CAD build for the part. Positions are in the model's coordinates, mm. Face numbers are marked on the shaded views. A direction names the side the tool comes from. Round coordinates to 2 decimals unless told otherwise and drop trailing zeros. Order: outer loops, then holes, each group sorted by start corner. A loop starts at its lowest first (then second) coordinate and runs counter-clockwise, first axis right, second up. Notation, with made-up numbers: (74.5, 4) - (86.5, 4) arc R12 cw to (86.5, 15) - close; hole circle Ø4 at (13.5, 20). An arc over 180 degrees is marked (long way). Use one line per item in the form item = value. Start each with the question number.
Autodesk Inventor part; units mm, degrees
ref_plane "YZ Plane" through (0, 0, 0) normal (1, 0, 0) x (0, 1, 0)
ref_plane "XZ Plane" through (0, 0, 0) normal (0, 1, 0) x (-1, 0, 0)
ref_plane "XY Plane" through (0, 0, 0) normal (0, 0, 1) x (1, 0, 0)
sketch "Sketch1" plane through (0, 0, 0) normal (0, 1, 0) x (-1, 0, 0)
  line L0 (28.5, 27) -> (-28.5, 27)
  line L1 (-28.5, 27) -> (-28.5, -27)
  line L2 (-28.5, -27) -> (28.5, -27)
  line L3 (28.5, -27) -> (28.5, 27)
  line L4 (28.5, 27) -> (-28.5, -27) construction
  line L5 (-28.5, 27) -> (28.5, -27) construction
  point P0 (0, 0)
  dimension "d0" = 57
  dimension "d1" = 54
extrude "Extrusion1" add sketch "Sketch1" along normal blind 1
sketch "Sketch2" plane through (0, 1, 0) normal (0, 1, 0) x (1, 0, 0)
  line L0 (-28.5, 27) -> (-28.5, -27)
  line L1 (28.5, -27) -> (28.5, 27)
  line L2 (-28.5, -27) -> (28.5, -27)
  line L3 (28.5, -27) -> (28.5, -26)
  line L4 (28.5, -26) -> (-28.5, -26)
  line L5 (-28.5, -26) -> (-28.5, -27)
  point P0 (0, 0)
  point P1 (-28.5, -26)
  dimension "d4" = 1
extrude "Extrusion2" add sketch "Sketch2" along normal blind 20
sketch "Sketch3" plane through (0, 1, 0) normal (0, 1, 0) x (1, 0, 0)
  line L0 (-28.5, 27) -> (-28.5, -27)
  line L1 (-28.5, -11) -> (28.5, -11) construction
  line L2 (28.5, -27) -> (28.5, 27)
  line L3 (28.5, -26) -> (-28.5, -26)
  line L4 (0, -26) -> (0, 22.5) construction
  circle A0 centre (-16.5, -11) radius 6.5
  circle A1 centre (16.5, -11) radius 6.5
  point P0 (0, 0)
  dimension "d7" = 15
  dimension "d8" = 13
  dimension "d9" = 12
extrude "Extrusion3" add sketch "Sketch3" along normal blind 3 draft -45
sketch "Sketch4" plane through (0, 0, 0) normal (0, -1, 0) x (1, 0, 0)
  circle A0 centre (16.5, 11) radius 3.5
  circle A1 centre (-16.5, 11) radius 3.5
  circle A2 centre (16.5, 11) radius 3.5
  circle A3 centre (-16.5, 11) radius 3.5
  point P0 (0, 0)
hole "Hole1" at (16.5, 0, 11) at (-16.5, 0, 11) direction (0, 1, 0) diameter 5.5118 end through all countersink diameter 12.7 countersink angle 90
fillet "Fillet1" radius 1 2 edges at (0, 1, 26) (0, 0, 27)
sketch "Sketch5" plane through (28.5, 0, 26) normal (1, 0, 0) x (0, 0, -1)
  line L0 (53, 1) -> (1, 1)
  arc A0 (53, 1) -> (46.65, 1) centre (49.825, 1) ccw
  line L1 (53, 0) -> (0, 0)
  arc A1 (46.65, 0) -> (53, 0) centre (49.825, 0) ccw
  point P0 (26, 0)
  dimension "d20" = 6.35
  dimension "d24" = 6.35
extrude "Extrusion4" add sketch "Sketch5" against normal up to surface (57 mm away)
fillet "Fillet2" radius 1 6 edges at (0, 1, -20.65) (0, 1, -27) (0, 0, -27) (28.5, 21, 26.5) (-28.5, 21, 26.5) (0, 0, -20.65)
equation "\"d24\" = d20"
properties part number "Handle V1"
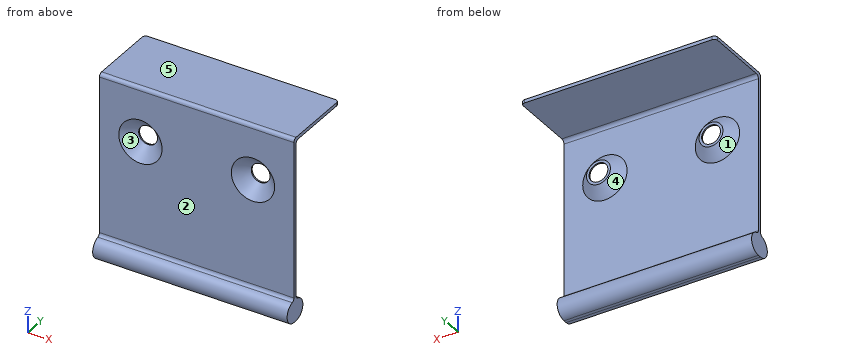
(1) Wall check: line 1 (Z direction, x = 16.5, y = 3.8); line 2 (X direction, y = 3.8, z = 11); line 3 (Z direction, x = -16.5, y = 3.9). Give the ranges that are in metal, low to high. Write a range as [from, to].
(2) Slice it at D-D (z = -2.5). Give the cut face in (x, y), and give its area (3 significant figures).
(3) Mould opens along X. For the marked faces 3, 4 and 5 say: pulls with the +X half, pulls with the -X half, needs draft (parallel to the pull), parting line crosses it, or undercut.
(4) Which spindle directions (+Z, -Z, +X, -X, +Y, -Y) get a long thin tool onto all of the face, cutting with end or side? Do the marked faces 1 and 2. Say none if no direction does.
(5) Slice it at C-C (x = -6.5). Give the cut face in (y, z) (3 decimals), and give its area (3 significant figures).
(6) Slice it at A-A (x = -16.5). Give the cut face in (y, z) (3 decimals), and give its area (3 significant figures).
(7) Slice it at B-B (z = 11). Give the cut face in (x, y).
(8) Flat gauge pins, fed straight in: P1, Ø3.5, axis at x = 18, z = 11, coming from the +Y side; P2, Ø1.5, axis at x = 4.5, z = -6, coming from the +Y side; P3, Ø4, axis at x = 16.5, z = -17.5, coming from the -Y side. Where does each tip first touch, or does it go through?
Results list:
q1.line_1 = [-25.32, -22.33], [7.3, 8.24], [13.76, 14.7], [26, 27]
q1.line_2 = [-20.2, -19.26], [-13.74, -12.8], [12.8, 13.74], [19.26, 20.2]
q1.line_3 = [-25.12, -22.53], [7.4, 8.24], [13.76, 14.6], [26, 27]
q2.outline = (-28.5, 0) - (28.5, 0) - (28.5, 1) - (-28.5, 1) - close
q2.area = 57.0 mm²
q3.face_3 = undercut
q3.face_4 = undercut
q3.face_5 = needs draft
q4.face_1 = +Y
q4.face_2 = +Z, +X, -X, -Y
q5.outline = (-0.76, -20.742) arc R3.175 ccw to (0, -27) - (1, -27) arc R3.175 ccw to (1.76, -20.742) arc R1 cw to (1, -19.772) - (1, 25) arc R1 cw to (2, 26) - (21, 26) - (21, 27) - (1, 27) arc R1 ccw to (0, 26) - (0, -19.772) arc R1 cw to start
q5.area = 106 mm²
q6.outline = (-0.76, -20.742) arc R3.175 ccw to (0, -27) - (1, -27) arc R3.175 ccw to (1.76, -20.742) arc R1 cw to (1, -19.772) - (1, 4.5) - (4, 7.5) - (4, 8.244) - (3.594, 8.244) - (0, 4.65) - (0, -19.772) arc R1 cw to start; (0, 17.35) - (3.594, 13.756) - (4, 13.756) - (4, 14.5) - (1, 17.5) - (1, 25) arc R1 cw to (2, 26) - (21, 26) - (21, 27) - (1, 27) arc R1 ccw to (0, 26) - close
q6.area = 101 mm²
q7.outline = (-28.5, 0) - (-22.85, 0) - (-19.26, 3.59) - (-19.26, 4) - (-20, 4) - (-23, 1) - (-28.5, 1) - close; (-13.74, 3.59) - (-10.15, 0) - (10.15, 0) - (13.74, 3.59) - (13.74, 4) - (13, 4) - (10, 1) - (-10, 1) - (-13, 4) - (-13.74, 4) - close; (19.26, 3.59) - (22.85, 0) - (28.5, 0) - (28.5, 1) - (23, 1) - (20, 4) - (19.26, 4) - close
q8.P1 = 4
q8.P2 = 1
q8.P3 = 0
